CAD build for the part. Positions are in the model's coordinates, mm. A direction names the side the tool comes from. Round coordinates to 2 decimals unless told otherwise and drop trailing zeros. Loops run counter-clockwise (first coordinate to the right, second up) from the corner with the lowest first, then second, coordinate; pieces in that order, holes last.
Autodesk Inventor part; units mm, degrees
ref_plane "YZ Plane" through (0, 0, 0) normal (1, 0, 0) x (0, 1, 0)
ref_plane "XZ Plane" through (0, 0, 0) normal (0, 1, 0) x (-1, 0, 0)
ref_plane "XY Plane" through (0, 0, 0) normal (0, 0, 1) x (1, 0, 0)
sketch "スケッチ1" plane through (0, 0, 0) normal (0, 1, 0) x (-1, 0, 0)
  line L0 (-40, -39) -> (40, -39)
  line L1 (40, -39) -> (40, 39)
  line L2 (40, 39) -> (-40, 39)
  line L3 (-40, 39) -> (-40, -39)
  line L4 (-40, -39) -> (40, 39) construction
  line L5 (40, -39) -> (-40, 39) construction
  point P0 (0, 0)
  dimension "d0" = 80
  dimension "d1" = 78
extrude "押し出し1" add sketch "スケッチ1" along normal blind 3
sketch "スケッチ2" plane through (0, 3, 0) normal (0, 1, 0) x (1, 0, 0)
  line L0 (34, 30) -> (-34, 30)
  line L1 (-34, 30) -> (-34, -30)
  line L2 (-34, -30) -> (34, -30)
  line L3 (34, -30) -> (34, 30)
  line L4 (34, 30) -> (-34, -30) construction
  line L5 (-34, 30) -> (34, -30) construction
  point P0 (0, 0)
  dimension "d4" = 68
  dimension "d5" = 60
hole "穴1" at (-34, 3, 30) at (34, 3, 30) at (34, 3, -30) at (-34, 3, -30) direction (0, -1, 0) diameter 5.2 depth 8 tip angle 118
sketch "スケッチ3" plane through (0, 3, 0) normal (0, 1, 0) x (1, 0, 0)
  line L0 (13.5, 25) -> (-13.5, 25)
  line L1 (-13.5, 25) -> (-13.5, -25)
  line L2 (-13.5, -25) -> (13.5, -25)
  line L3 (13.5, -25) -> (13.5, 25)
  line L4 (13.5, 25) -> (-13.5, -25) construction
  line L5 (-13.5, 25) -> (13.5, -25) construction
  point P0 (0, 0)
  dimension "d13" = 27
  dimension "d14" = 50
hole "穴2" at (-13.5, 3, 25) at (13.5, 3, 25) at (13.5, 3, -25) at (-13.5, 3, -25) direction (0, -1, 0) diameter 5.3 depth 8 tip angle 118 countersink diameter 10 countersink angle 90
sketch "スケッチ5" plane through (0, 0, 0) normal (0, -1, 0) x (1, 0, 0)
  line L0 (74, 39) -> (-74, 39)
  line L1 (-74, 39) -> (-74, -39)
  line L2 (-74, -39) -> (74, -39)
  line L3 (74, -39) -> (74, 39)
  circle A0 centre (13.5, -25) radius 2.65
  circle A1 centre (13.5, -25) radius 2.65
  circle A2 centre (-13.5, 25) radius 2.65
  circle A3 centre (13.5, 25) radius 2.65
  circle A4 centre (-13.5, -25) radius 2.65
  circle A5 centre (34, -30) radius 2.6
  circle A6 centre (-34, 30) radius 2.6
  circle A7 centre (34, 30) radius 2.6
  circle A8 centre (-34, -30) radius 2.6
  line L4 (-40, -39) -> (-40, 39)
  line L5 (40, -39) -> (-40, -39)
  line L6 (40, 39) -> (40, -39)
  line L7 (-40, 39) -> (40, 39)
  point P0 (0, 0)
  point P1 (-40, 39)
  dimension "d28" = 40
  dimension "d29" = 40
extrude "押し出し3" add sketch "スケッチ5" against normal up to surface (3 mm away) contours L3 L2 L6 L0 | L4 L2 L1 L0
sketch "スケッチ6" plane through (0, 0, 0) normal (0, -1, 0) x (1, 0, 0)
  circle A0 centre (13.5, -25) radius 2.65
  circle A1 centre (-13.5, 25) radius 2.65
  circle A2 centre (13.5, 25) radius 2.65
  circle A3 centre (-13.5, -25) radius 2.65
  circle A4 centre (34, -30) radius 2.6
  circle A5 centre (-34, 30) radius 2.6
  circle A6 centre (34, 30) radius 2.6
  circle A7 centre (-34, -30) radius 2.6
  line L0 (-74, -39) -> (74, -39)
  line L1 (74, -39) -> (74, 39)
  line L2 (74, 39) -> (-74, 39)
  line L3 (-74, 39) -> (-74, -39)
  line L4 (74, -39) -> (44, -39)
  line L5 (44, -39) -> (44, -42)
  line L6 (44, -42) -> (74, -42)
  line L7 (74, -42) -> (74, -39)
  line L8 (-74, 39) -> (-74, -39)
  line L9 (-74, -39) -> (-44, -39)
  line L10 (-44, -39) -> (-44, -42)
  line L11 (-44, -42) -> (-74, -42)
  line L12 (-74, -42) -> (-74, -39)
  line L13 (44, -42) -> (-44, -42)
  line L14 (-44, -42) -> (-44, -39)
  line L15 (-44, -39) -> (44, -39)
  line L16 (44, -39) -> (44, -42)
  point P0 (0, 0)
  dimension "d33" = 30
  dimension "d34" = 30
  dimension "d49" = 3
extrude "押し出し5" add sketch "スケッチ6" against normal up to surface (3 mm away) contours L0 L10 L11 L12 | L0 L7 L6 L5
sketch "スケッチ8" plane through (74, 0, -42) normal (0, 0, -1) x (-1, 0, 0)
  line L0 (30, 0) -> (0, 0)
  line L1 (0, 0) -> (0, -42)
  line L2 (0, -42) -> (30, -42)
  line L3 (30, -42) -> (30, 0)
edge flange "フランジ2" height 45 angle 90 thickness 3 bend radius 3 thickness toward (0, 0, -1) relief straight relief width 3 relief depth 1.5 corner gap 3 corner form 0 edges at (59, 0, -42) (-59, 0, -42) wall of the first edge with corners at (44, 0, -42) (74, 0, -42) (74, -42, -42) (44, -42, -42)
bend "曲げ2"
corner "コーナー2"
sketch "スケッチ9" plane through (-44, -42, -45) normal (0, 0, -1) x (-1, 0, 0)
  line L0 (30, 39) -> (0, 39)
  line L1 (0, 0) -> (0, 39)
  line L2 (30, 0) -> (0, 0)
  line L3 (30, 39) -> (30, 0)
  line L4 (-88, 39) -> (-118, 39)
  line L5 (-118, 0) -> (-118, 39)
  line L6 (-88, 0) -> (-118, 0)
  line L7 (-88, 39) -> (-88, 0)
  point P0 (-44, 42)
  point P1 (15, 10)
  point P2 (-103, 10)
  dimension "d62" = 10
  dimension "d63" = 15
  dimension "d64" = 15
hole "穴3" at (-59, -32, -45) at (59, -32, -45) direction (0, 0, 1) diameter 6.2 depth 3 tip angle 118
fillet "フィレット3" radius 2 4 edges at (-74, -42, -43.5) (-44, -42, -43.5) (44, -42, -43.5) (74, -42, -43.5)
equation "\"d28\" = d29"
equation "\"d70\" = Thickness"
equation "\"d38\" = Thickness"
equation "\"d52\" = BendReliefWidth"
equation "\"d53\" = BendReliefDepth"
equation "\"d54\" = MinimumRemnant"
equation "\"d55\" = TransitionRadius"
equation "\"d58\" = BendRadius"
equation "\"d59\" = CornerReliefSize"
equation "\"d60\" = GapSize"
equation "\"d61\" = JacobiRadiusSize"
equation "\"BendRadius\" = Thickness"
equation "\"BendReliefWidth\" = Thickness"
equation "\"BendReliefDepth\" = 0.5 * Thickness"
equation "\"CornerReliefSize\" = 4 * Thickness"
equation "\"MinimumRemnant\" = 2 * Thickness"
equation "\"TransitionRadius\" = BendRadius"
equation "\"JacobiRadiusSize\" = Thickness"
equation "\"GapSize\" = Thickness"
properties part number "CCM_Mount_F"
Item 1: 3-axis set-ups, long thin cutter, end or side, ignore diameter. For faces 1 (the flat face through (-59, -22, -42)), 2 (the cylindrical face through (32.243, 1.479, 28.084)), 3 (the flat face through (44, -19, -43)), 4 (the flat face through (74, 1, -16)): which of +Z, -Z, +X, -X, +Y, -Y reach the whole face in a straight line?
Answers follow:
face 1: +Z, +X, -X, -Y
face 2: +Y, -Y
face 3: -Z, +Y, -Y
face 4: +Z, -Z, +X, +Y, -Y
Item 2: Cut at C-C, the plane z = -25. Give the cut face in (x, y).
Answers follow:
outline: (-74, 0) - (-16.15, 0) - (-16.15, 0.65) - (-18.5, 3) - (-74, 3) - close; (-10.85, 0) - (10.85, 0) - (10.85, 0.65) - (8.5, 3) - (-8.5, 3) - (-10.85, 0.65) - close; (16.15, 0) - (74, 0) - (74, 3) - (18.5, 3) - (16.15, 0.65) - close
Item 3: Flat gauge pins, fed straight in: P1, Ø7, axis at x = -34, z = -30, coming from the -Y side; P2, Ø1.5, axis at x = 9.5, y = 1.5, coming from the -Z side; P3, Ø4.5, axis at x = 34, z = -30, coming from the -Y side; P4, Ø15, axis at x = 55.5, y = -31.5, coming from the +Z side. Where does each tip first touch, or does it go through?
Answers follow:
P1: stops at y = 0
P2: stops at z = -39
P3: passes through
P4: stops at z = -42
Item 4: Two-plate mould, pull along X, no slides. Class faces 5 (the flat face through (1, 1, -39)), 6 (the flat face through (-74, 1, -15)), 7 (the flat face through (-59, -23, -45)): released by +X, released by -X, zero draft, split by the parting line, or undercut.
Answers follow:
face 5: undercut
face 6: released by -X
face 7: zero draft
Item 5: Cut at B-B, the plane y = -32. Give the cut face in (x, z).
Answers follow:
outline: (-74, -45) - (-62.1, -45) - (-62.1, -42) - (-74, -42) - close; (-55.9, -45) - (-44, -45) - (-44, -42) - (-55.9, -42) - close; (44, -45) - (55.9, -45) - (55.9, -42) - (44, -42) - close; (62.1, -45) - (74, -45) - (74, -42) - (62.1, -42) - close
Item 6: Cut at A-A, the plane x = 13.5. Give the cut face in (y, z).
Answers follow:
outline: (0, -39) - (3, -39) - (3, -30) - (0.65, -27.65) - (0, -27.65) - close; (0, -22.35) - (0.65, -22.35) - (3, -20) - (3, 20) - (0.65, 22.35) - (0, 22.35) - close; (0, 27.65) - (0.65, 27.65) - (3, 30) - (3, 39) - (0, 39) - close
Item 7: Cut at D-D, the plane x = -59. Give the cut face in (y, z).
Answers follow:
outline: (-42, -45) - (-35.1, -45) - (-35.1, -42) - (-42, -42) - close; (-28.9, -45) - (-3, -45) arc R6 ccw to (3, -39) - (3, 39) - (0, 39) - (0, -39) arc R3 cw to (-3, -42) - (-28.9, -42) - close
Item 8: Probe line 1 (X direction, y = 2.1, z = -30); line 2 (Z direction, x = -34, y = 1.4); line 3 (Z direction, x = -13.5, y = 0.55). List the from-to ranges inside material, lowest first.
Answers follow:
line 1: x = -74 to -36.6, -31.4 to 31.4, 36.6 to 74
line 2: z = -39 to -32.6, -27.4 to 27.4, 32.6 to 39
line 3: z = -39 to -27.65, -22.35 to 22.35, 27.65 to 39
